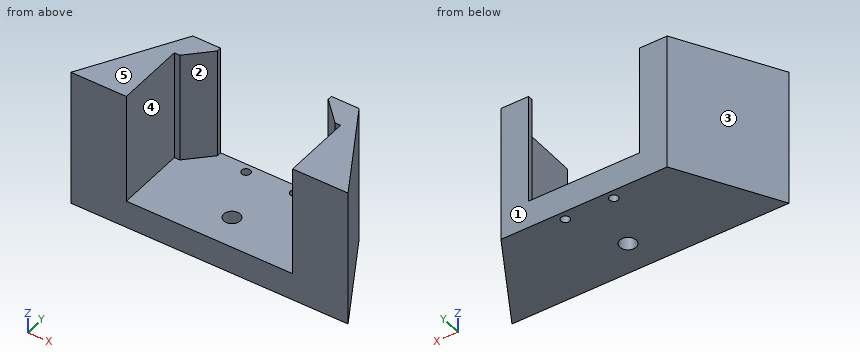
Autodesk Inventor part; units mm, degrees
ref_plane "YZ Plane" through (0, 0, 0) normal (1, 0, 0) x (0, 1, 0)
ref_plane "XZ Plane" through (0, 0, 0) normal (0, 1, 0) x (-1, 0, 0)
ref_plane "XY Plane" through (0, 0, 0) normal (0, 0, 1) x (1, 0, 0)
sketch "Sketch1" plane through (0, 0, 0) normal (0, 0, 1) x (1, 0, 0)
  line L0 (0, 0) -> (100, 0)
  line L1 (0, 0) -> (20, 34.641)
  line L2 (0, 0) -> (40, 0) construction
  line L3 (100, 0) -> (80, 34.641)
  line L4 (100, 0) -> (140, 0) construction
  line L5 (20, 34.641) -> (80, 34.641)
  dimension "d0" = 100
  dimension "d1" = 40
  dimension "d2" = 60
  dimension "d3" = 40
  dimension "d4" = 120
extrude "Extrusion1" add sketch "Sketch1" along normal blind 30
sketch "Sketch2" plane through (0, 0, 30) normal (0, 0, 1) x (1, 0, 0)
  line L0 (0, 0) -> (100, 0)
  line L1 (20, 0) -> (80, 0)
  line L2 (80, 0) -> (80, 25)
  line L3 (80, 25) -> (20, 25)
  line L4 (20, 25) -> (20, 0)
  dimension "d7" = 60
  dimension "d8" = 25
  dimension "d9" = 20
extrude "Extrusion2" cut sketch "Sketch2" against normal blind 20
ref_plane "Work Plane1" through (0, -10, 0) normal (0, -1, 0) x (1, 0, 0)
sketch "Sketch4" plane through (20, 34.641, 0) normal (0, 1, 0) x (1, 0, 0)
  line L0 (60, -10) -> (0, -10)
  line L1 (10, -10) -> (50, -10)
  line L2 (50, -10) -> (50, -35)
  line L3 (50, -35) -> (10, -35)
  line L4 (10, -35) -> (10, -10)
  point P0 (-20, 0)
  point P1 (30, -10)
  point P2 (50, -10)
  dimension "d19" = 40
  dimension "d20" = 25
  dimension "d21" = 20
extrude "Extrusion4" cut sketch "Sketch4" against normal through all
chamfer "Chamfer1" distance 8 angle 45 1 edges at (30, 25, 20)
chamfer "Chamfer2" distance 8 angle 45 1 edges at (70, 25, 20)
sketch "Sketch6" plane through (0, 0, 30) normal (0, 0, 1) x (1, 0, 0)
  line L0 (30, 33) -> (22, 25)
  line L1 (30, 33) -> (30, 34.641)
  line L2 (30, 34.641) -> (20, 34.641)
  line L3 (20, 34.641) -> (0, 0)
  line L4 (0, 0) -> (20, 0)
  line L5 (20, 0) -> (20, 25)
  line L6 (20, 25) -> (22, 25)
  line L7 (78, 25) -> (70, 33)
  line L8 (78, 25) -> (80, 25)
  line L9 (80, 25) -> (80, 0)
  line L10 (80, 0) -> (100, 0)
  line L11 (100, 0) -> (80, 34.641)
  line L12 (80, 34.641) -> (70, 34.641)
  line L13 (70, 34.641) -> (70, 33)
extrude "Extrusion6" add sketch "Sketch6" along normal blind 20
sketch "Sketch8" plane through (0, 0, 0) normal (0, 0, -1) x (-1, 0, 0)
  line L0 (-39.0839, 36.891) -> (-43.0739, 36.891)
  line L1 (-43.0739, 48.241) -> (-43.0739, 36.891)
  line L2 (-57.1939, 48.241) -> (-43.0739, 48.241)
  line L3 (-57.1939, 48.241) -> (-57.1939, 36.891)
  line L4 (-57.1939, 36.891) -> (-61.1839, 36.891)
  line L5 (-61.1839, 36.891) -> (-61.1839, 5.041)
  line L6 (-56.3339, 0.191) -> (-43.9339, 0.191)
  line L7 (-39.0839, 5.041) -> (-39.0839, 36.891)
  line L8 (-52.9432, 43.5972) -> (-47.3245, 43.5972)
  line L9 (-52.9432, 43.5972) -> (-52.9432, 44.1479)
  line L10 (-52.4839, 44.6341) -> (-52.9432, 44.1479)
  line L11 (-52.4839, 44.6341) -> (-47.7839, 44.6341)
  line L12 (-47.3245, 44.1479) -> (-47.7839, 44.6341)
  line L13 (-47.3245, 44.1479) -> (-47.3245, 43.5972)
  circle A0 centre (-58.8839, 31.541) radius 1.575
  circle A1 centre (-41.3839, 31.541) radius 1.575
  circle A2 centre (-50.1339, 11.541) radius 2.75
  circle A3 centre (-50.1339, 11.541) radius 2.95
  arc A4 (-61.1839, 5.041) -> (-56.3339, 0.191) centre (-56.3339, 5.041) ccw
  arc A5 (-43.9339, 0.191) -> (-39.0839, 5.041) centre (-43.9339, 5.041) ccw
  circle A6 centre (-50.1339, 11.541) radius 2.75
  circle A7 centre (-41.6839, 2.741) radius 0.75
  circle A8 centre (-58.5839, 2.741) radius 0.75
  circle A9 centre (-40.7939, 35.041) radius 1
  circle A10 centre (-59.4739, 35.041) radius 1
  circle A11 centre (-58.8839, 31.541) radius 1.575
  circle A12 centre (-41.3839, 31.541) radius 1.575
  point P0 (0, 0)
extrude "Extrusion8" cut sketch "Sketch8" against normal up to surface (10 mm away) contours A0 | A1 | A2 | A3
properties part number "Wheel_well"
Check sheet for the modelled part. Datum: model origin and axes. Units: mm. Face numbers are marked on the shaded views. A direction names the side the tool comes from. Round coordinates to 2 decimals unless told otherwise and drop trailing zeros. Write each loop counter-clockwise with the first axis right and the second up, starting at its lowest first coordinate (ties: lowest second). Pieces come first, ordered by that corner, then holes. Notation, with made-up numbers: (56, 87) - (83, 87) arc R17 cw to (83, 105) - close; hole circle Ø8 at (75, 88). An arc over 180 degrees is marked (long way). Return JSON: item names as keys, results as strings.
Q1. Draft check along X on the marked faces 1, 2 and 3. Enter one of: released by +X, released by -X, zero draft, split by the parting line, or undercut.
Returned:
{"face 1": "zero draft", "face 2": "undercut", "face 3": "released by -X"}
Q2. Depth check by flat-ended pin: P1, Ø4, axis at x = 27.5, y = 14.5, coming from the +Z side; P2, Ø1.8, axis at y = 34, z = 35.5, coming from the +X side; P3, Ø0.5, axis at y = 33.5, z = 27, coming from the -X side. Enter the tip coordinate at first touch or a pass-through.
Returned:
{"P1": "stops at z = 10", "P2": "stops at x = 80.89", "P3": "stops at x = 19.2"}
Q3. Cross-section at B-B (x = 41). Record the boundary of the cut face in (y, z).
Returned:
{"outline": "(0, 0) - (30.01, 0) - (30.01, 10) - (0, 10) - close; (33.07, 0) - (34.64, 0) - (34.64, 10) - (33.07, 10) - close"}
Q4. Cross-section at D-D (z = 5). Record the boundary of the cut face in (x, y) (3 decimals).
Returned:
{"outline": "(0, 0) - (100, 0) - (80, 34.641) - (20, 34.641) - close; hole circle Ø3.15 at (41.384, 31.541); hole circle Ø5.9 at (50.134, 11.541); hole circle Ø3.15 at (58.884, 31.541)"}
Q5. Cross-section at C-C (y = 20). Record the boundary of the cut face in (x, z), then the cut area to 3 significant figures.
Returned:
{"outline": "(11.55, 0) - (88.45, 0) - (88.45, 50) - (80, 50) - (80, 10) - (20, 10) - (20, 50) - (11.55, 50) - close", "area": "1,450 mm²"}
Q6. Scan lines: L1, parallel to Z at x = 35.5, y = 15; L2, parallel to X at y = 32.5, z = 27; L3, parallel to X at y = 21, z = 14.5. Record each from-to range of solid material in increasing order. Write a range as from..to.
Returned:
{"L1": "z = 0..10", "L2": "x = 18.76..29.5, 70.5..81.24", "L3": "x = 12.12..20, 80..87.88"}
Q7. Cross-section at A-A (z = 11). Record the boundary of the cut face in (x, y).
Returned:
{"outline": "(0, 0) - (20, 0) - (20, 25) - (22, 25) - (30, 33) - (30, 34.64) - (20, 34.64) - close; (70, 33) - (78, 25) - (80, 25) - (80, 0) - (100, 0) - (80, 34.64) - (70, 34.64) - close"}
Q8. Access from +Z, -Z, +X, -X, +Y, -Y to the whole of each face (thin tool, end or side, straight path). Record for the marked faces 4 and 5.
Returned:
{"face 4": "+Z, -Y", "face 5": "+Z, +X, -X, +Y, -Y"}
